Input: part model. Units: mm. Frame: model coordinates. Give positions to 0.01 mm unless a question says otherwise; leave off trailing zeros. Loops run counter-clockwise (first coordinate to the right, second up) from the corner with the lowest first, then second, coordinate; pieces in that order, holes last. Notation, with made-up numbers: M -15.75,53 L 37.25,53 A10 ccw 37.25,64 Z; hole C -17.5,76 d3. An arc over 180 degrees is marked long. Answer as a JSON object with one key per item and string values. Group by question number.
1) Section query D-D on x = 39. Count the separate pieces of the cut face and the enclosed holes in it, plus the area to 3 significant figures.
2) Section query B-B on x = 53.5. Return loops of the section in (y, z).
3) Section query C-C on x = 16.5. Return loops of the section in (y, z), plus the area to 3 significant figures.
4) First-contact query: P1, Ø4.5, axis at x = 6.13, y = -8.44, coming from the -Z side. Flat tip, straight axial feed; report the tip coordinate or a pass-through.
5) Ray query, L1, parallel to X at y = 16, z = 1.1; L2, parallel to X at y = 36, z = 2; L3, parallel to Y at x = 20.5, z = 1.7. Return the intervals inside material, ascending.
6) Section query A-A on y = 15. Return loops of the section in (x, z), plus the area to 3 significant figures.
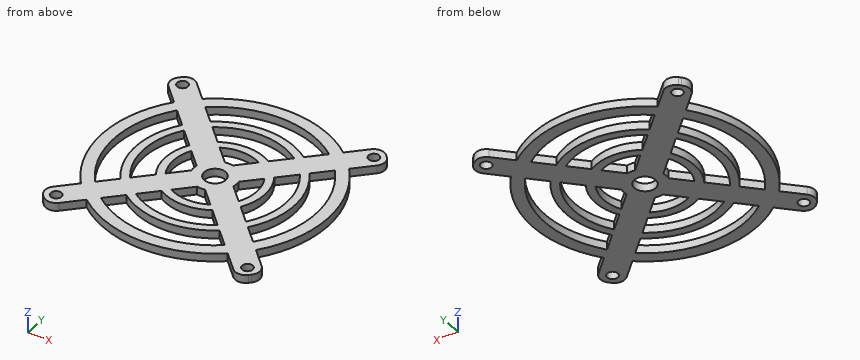
Autodesk Inventor part; units mm, degrees
ref_plane "YZ Plane" through (0, 0, 0) normal (1, 0, 0) x (0, 1, 0)
ref_plane "XZ Plane" through (0, 0, 0) normal (0, 1, 0) x (-1, 0, 0)
ref_plane "XY Plane" through (0, 0, 0) normal (0, 0, 1) x (1, 0, 0)
sketch "Szkic1" plane through (0, 0, 0) normal (0, 0, 1) x (1, 0, 0)
  circle A0 centre (41.8843, 27.3116) radius 37.5
  circle A1 centre (41.8843, 27.3116) radius 42
  circle A2 centre (41.8843, 27.3116) radius 29.5
  circle A3 centre (41.8843, 27.3116) radius 26.5
  circle A4 centre (41.8843, 27.3116) radius 18.5
  circle A5 centre (41.8843, 27.3116) radius 15.5
  circle A6 centre (41.8843, 27.3116) radius 8
  line L0 (0.1239, 62.7081) -> (6.4879, 69.072)
  line L1 (83.6448, 62.7081) -> (77.2808, 69.072)
  line L2 (77.2808, -14.4488) -> (83.6448, -8.0848)
  line L3 (0.1239, -8.0848) -> (6.4879, -14.4488)
  line L4 (0.1239, 62.7081) -> (77.2808, -14.4488)
  line L5 (6.4879, 69.072) -> (83.6448, -8.0848)
  line L6 (0.1239, -8.0848) -> (77.2808, 69.072)
  line L7 (6.4879, -14.4488) -> (83.6448, 62.7081)
  point P0 (0, 0)
  point P1 (0, 0)
  point P2 (6.1343, 63.0616)
  point P3 (77.6343, 63.0616)
  point P4 (77.6343, -8.4384)
  point P5 (6.1343, -8.4384)
  dimension "d0" = 75
  dimension "d1" = 35.75
  dimension "d2" = 35.75
  dimension "d3" = 35.75
  dimension "d4" = 35.75
  dimension "d5" = 35.75
  dimension "d6" = 35.75
  dimension "d7" = 35.75
  dimension "d8" = 35.75
  dimension "d9" = 4.5
  dimension "d20" = 8
  dimension "d21" = 3
  dimension "d22" = 8
  dimension "d23" = 3
  dimension "d24" = 16
  dimension "d33" = 4
  dimension "d34" = 4
  dimension "d35" = 4
  dimension "d36" = 4
extrude "Wyciągnięcie proste1" add sketch "Szkic1" along normal blind 3 contours A0 L7 A1 L5 | L7 A2 L6 A0 | A0 L6 A1 L7 | L5 A1 L4 A0 | A0 L4 A2 L5 | A0 L5 A1 L6 | L7 A3 L6 A2 | A2 L5 A3 L7 | A1 L6 L1 L7 | L4 A1 L7 A0 | A2 L4 A3 L5 | L5 L2 L4 A1 | L5 A2 L4 A0 | A0 L4 A1 L5 | L6 A3 L5 A2 | L7 A4 L6 A3 | L7 A1 L6 A0 | A0 L6 A2 L7 | A2 L7 A3 L4 | A3 L4 A4 L5 | A0 L6 A1 L4 | A1 L4 L0 L5 | L5 A3 L4 A2 | L7 A5 L6 A4 | A4 L5 A5 L7 | L7 L3 L6 A1 | A2 L6 A3 L7 | A4 L4 A5 L5 | L4 A3 L6 A2 | L5 A4 L4 A3 | L6 A5 L5 A4 | L7 A6 L6 A5 | A3 L6 A4 L7 | A4 L7 A5 L4 | A5 L4 A6 L5 | L5 A5 L4 A4 | L7 L5 L6 A6 | A6 L5 L7 | A4 L6 A5 L7 | A6 L4 L7 L5 | L4 A5 L6 A4 | L5 A6 L4 A5 | L6 L5 A6 | L7 L4 L6 L5 | A5 L6 A6 L7 | A6 L7 L4 | L5 L6 L4 A6 | L7 A6 L6 L4 | L4 L6 A6
hole "Otwór1" at (6.1343, -8.4384, 0) at (77.6343, -8.4384, 0) at (77.6343, 63.0616, 0) at (6.1343, 63.0616, 0) direction (0, 0, 1) diameter 4 end through all
fillet "Zaokrąglenie1" radius 4 8 edges at (6.4879, -14.4488, 1.5) (0.1239, -8.0848, 1.5) (77.2808, -14.4488, 1.5) (83.6448, -8.0848, 1.5) (83.6448, 62.7081, 1.5) (77.2808, 69.072, 1.5) (0.1239, 62.7081, 1.5) (6.4879, 69.072, 1.5)
hole "Otwór2" at (41.8843, 27.3116, 0) direction (0, 0, 1) diameter 8 depth 8 tip angle 118
equation "\"d17\" = d16"
equation "\"d18\" = d16"
equation "\"d19\" = d16"
properties part number "3DP_PLA_Controller_Case_Fan_Grill"
Output:
{
 "1": {"separate pieces": "8", "enclosed holes": "0", "area": "102 mm^2"},
 "2": {"outline": "M -13.05,0 L -8.34,0 L -8.34,3 L -13.05,3 Z; M 0.19,0 L 3.49,0 L 3.49,3 L 0.19,3 Z; M 9.33,0 L 22.06,0 L 22.06,3 L 9.33,3 Z; M 32.56,0 L 45.29,0 L 45.29,3 L 32.56,3 Z; M 51.13,0 L 54.43,0 L 54.43,3 L 51.13,3 Z; M 62.97,0 L 67.67,0 L 67.67,3 L 62.97,3 Z"},
 "3": {"outline": "M -6.15,0 L 8.29,0 L 8.29,3 L -6.15,3 Z; M 12.28,0 L 19.7,0 L 19.7,3 L 12.28,3 Z; M 34.92,0 L 42.34,0 L 42.34,3 L 34.92,3 Z; M 46.33,0 L 60.77,0 L 60.77,3 L 46.33,3 Z", "area": "131 mm^2"},
 "4": {"P1": "stops at z = 0"},
 "5": {"L1": "x = 1.44 to 6.13, 14.64 to 17.92, 24.21 to 36.94, 46.83 to 59.56, 65.85 to 69.13, 77.64 to 82.33", "L2": "x = 0.79 to 5.4, 13.69 to 16.85, 25.55 to 39.56, 44.21 to 58.22, 66.92 to 70.08, 78.36 to 82.98", "L3": "y = -8.84 to -3.49, -0.44 to 12.29, 42.33 to 55.06, 58.12 to 63.46"},
 "6": {"outline": "M 1.73,0 L 6.46,0 L 6.46,3 L 1.73,3 Z; M 15.08,0 L 18.42,0 L 18.42,3 L 15.08,3 Z; M 23.21,0 L 35.94,0 L 35.94,3 L 23.21,3 Z; M 47.83,0 L 60.56,0 L 60.56,3 L 47.83,3 Z; M 65.35,0 L 68.69,0 L 68.69,3 L 65.35,3 Z; M 77.31,0 L 82.04,0 L 82.04,3 L 77.31,3 Z", "area": "125 mm^2"}
}
